from build123d import *

# Parameters (mm, degrees)
SKETCH1_W                    = 1126.47095
SKETCH1_H                    = 71.4375
BASE_FLANGE1_DEPTH           = 3.2639
EDGE_FLANGE2_DEPTH           = 71.4375
F_10_0_1935_DIAMETER_HOLE1_D = 4.9149
LPATTERN1_COUNT              = 6
LPATTERN1_PITCH              = 215.265
F_10_0_1935_DIAMETER_HOLE2_D = 4.9149
FILLET1_R                    = 6.35


# Sheet-metal steps are written as plain solids
with BuildPart() as part:
    # Sketch1 → Base-Flange1 (new body)
    with BuildSketch(Plane(origin=(0, 0, 0), x_dir=(1, 0, 0), z_dir=(0, 1, 0))):
        with Locations((-563.235475, 0)):
            Rectangle(SKETCH1_W, SKETCH1_H)
    extrude(amount=-BASE_FLANGE1_DEPTH)

    # Edge-Flange2 section (across the edge) → Edge-Flange2 (add)
    with BuildSketch(Plane(origin=(1.27, 0, 35.71875), x_dir=(-1, 0, 0), z_dir=(0, 0, -1))):
        with BuildLine():
            Line((-3.2639, 1.27), (-3.2639, 28.4861))
            Line((-3.2639, 28.4861), (0, 28.4861))
            Line((0, 28.4861), (0, 1.27))
            ThreePointArc((0, 1.27), (0.371974388, 0.371974388), (1.27, 0))
            Line((1.27, 0), (1.27, -3.2639))
            ThreePointArc((1.27, -3.2639), (-1.935951435, -1.935951435), (-3.2639, 1.27))
        make_face()
    extrude(amount=EDGE_FLANGE2_DEPTH)

    # #10 (0.1935) Diameter Hole1 (through all)
    with Locations(Plane(origin=(0, 0, 0), x_dir=(1, 0, 0), z_dir=(0, 1, 0))):
        with Locations((-16.1036, 24.60625), (-16.1036, -24.60625)):
            f_10_0_1935_diameter_hole1 = Hole(F_10_0_1935_DIAMETER_HOLE1_D / 2)

    # LPattern1: #10 (0.1935) Diameter Hole1 ×6
    with Locations(*[(-i * LPATTERN1_PITCH, 0, 0) for i in range(1, LPATTERN1_COUNT)]):
        add(f_10_0_1935_diameter_hole1, mode=Mode.SUBTRACT)

    # #10 (0.1935) Diameter Hole2 (through all)
    with Locations(Plane.ZY.offset(-1.27)):
        with Locations((-23.8125, 19.05), (23.8125, 19.05)):
            Hole(F_10_0_1935_DIAMETER_HOLE2_D / 2)

    # Fillet1
    fillet1_edges = [part.edges().sort_by_distance(p)[0] for p in [
        (2.90195, 28.4861, 35.71875),
        (2.90195, 28.4861, -35.71875),
        (-1126.47095, -1.63195, -35.71875),
        (-1126.47095, -1.63195, 35.71875),
    ]]
    fillet(fillet1_edges, radius=FILLET1_R)


solid = part.part
Can you work these out from the model? Positions are in its coordinate system, mm. Give positions to 0.01 mm unless a question says otherwise; leave off trailing zeros. Loops run counter-clockwise (first coordinate to the right, second up) from the corner with the lowest first, then second, coordinate; pieces in that order, holes last. Notation, with made-up numbers: (62, 44) - (89, 44) arc R31 ccw to (89, 79) - close; hole circle Ø1 at (-13, 9). An arc over 180 degrees is marked (long way). Answer as a JSON object with one key per item and string values.
Q1. If we mould it in two halves opening along Y, with no side actions, what happens to faces 1 (the flat face through (-571, -3.264, -1)), 2 (the flat face through (1.27, 15, 1)), 3 (the flat face through (-571, 0, -1))? For each: pulls with the +Y half, pulls with the -Y half, needs draft (parallel to the pull), parting line crosses it, or undercut.
Geometry says:
{"face 1": "pulls with the -Y half", "face 2": "needs draft", "face 3": "pulls with the +Y half"}
Q2. Imagine slicing it at B-B on x = -708. Write out the boundary of the cut face in (y, z).
Geometry says:
{"outline": "(-3.26, -35.72) - (0, -35.72) - (0, 35.72) - (-3.26, 35.72) - close"}
Q3. If I drill on L1, parallel to Z at x = 2, y = 19; L2, parallel to Y at x = -202.5, z = 17; L3, parallel to X at y = 15.5, z = -12, over which ranges is the centre line in solid material (lowest first)?
Geometry says:
{"L1": "-35.72 to -26.27, -21.36 to 21.36, 26.27 to 35.72", "L2": "-3.26 to 0", "L3": "1.27 to 4.53"}
Q4. Imagine slicing it at A-A on z = 6. Write out the boundary of the cut face in (x, y).
Geometry says:
{"outline": "(-1126.47, -3.26) - (0, -3.26) arc R4.53 ccw to (4.53, 1.27) - (4.53, 28.49) - (1.27, 28.49) - (1.27, 1.27) arc R1.27 cw to (0, 0) - (-1126.47, 0) - close"}
Q5. Will these pins go through, and if not, where does the flat tip stop? P1, Ø1.5, axis at y = 10.5, z = -24.5, coming from the -X side; P2, Ø12, axis at x = -286.5, z = -25, coming from the +Y side.
Geometry says:
{"P1": "x = 1.27", "P2": "y = 0"}
